Geometry check sheet. Reference: the model listing, model coordinates, mm. Round coordinates to 2 decimals unless told otherwise and drop trailing zeros. Write each loop counter-clockwise with the first axis right and the second up, starting at its lowest first coordinate (ties: lowest second). Pieces come first, ordered by that corner, then holes. Notation, with made-up numbers: (-35, 36.5) -> (-29, 36.5) arc R16 ccw to (-29, 66.5) -> close; hole circle Ø7 at (-27, 69.25). An arc over 180 degrees is marked (long way). One line per question, with ' | ' between items.
```python
from build123d import *

# Parameters (mm, degrees)
EXTRUDE_THIN1_START = 1
EXTRUDE_THIN1_DEPTH = 6.35


with BuildPart() as part:
    # Sketch1 → Extrude-Thin1 (new body)
    with BuildSketch(Plane.XY.offset(EXTRUDE_THIN1_START)):
        with BuildLine():
            Line((388.165618503, 2.23097434), (388.165618503, 5.41097434))
            ThreePointArc((388.165618503, 5.41097434), (388.136623681, 5.481389287), (388.066453208, 5.510970857))
            Line((388.066453208, 5.510970857), (0.059901443, 8.749794959))
            ThreePointArc((0.059901443, 8.749794959), (-8.749999578, 0.002718342), (0.054464874, -8.749830488))
            Line((0.054464874, -8.749830488), (487.776522402, -5.713917899))
            ThreePointArc((487.776522402, -5.713917899), (493.304398035, -0.153253749), (487.779978506, 5.410843992))
            Line((487.779978506, 5.410843992), (428.265786749, 5.510974199))
            ThreePointArc((428.265786749, 5.510974199), (428.194967334, 5.481744477), (428.165618503, 5.41097434))
            Line((428.165618503, 5.41097434), (428.165618503, 2.23097434))
            Line((428.165618503, 2.23097434), (427.665618503, 2.23097434))
            Line((427.665618503, 2.23097434), (427.665618503, 5.41097434))
            ThreePointArc((427.665618503, 5.410974341), (427.841711488, 5.835595162), (428.266627977, 6.010973491))
            Line((428.266627977, 6.010973491), (487.78208283, 5.91084116))
            ThreePointArc((487.78208283, 5.91084116), (493.804398179, -0.15274976), (487.77963468, -6.213908213))
            Line((487.77963468, -6.213908213), (0.057577153, -9.249820802))
            ThreePointArc((0.057577153, -9.249820802), (-9.249999493, 0.003063934), (0.063704889, 9.249780629))
            Line((0.063704889, 9.249780629), (388.070626735, 6.010953438))
            ThreePointArc((388.070626735, 6.010953438), (388.491649569, 5.833464021), (388.665618503, 5.410974341))
            Line((388.665618503, 5.410974341), (388.665618503, 2.23097434))
            Line((388.665618503, 2.23097434), (388.165618503, 2.23097434))
        make_face()
    extrude(amount=EXTRUDE_THIN1_DEPTH)


solid = part.part
```
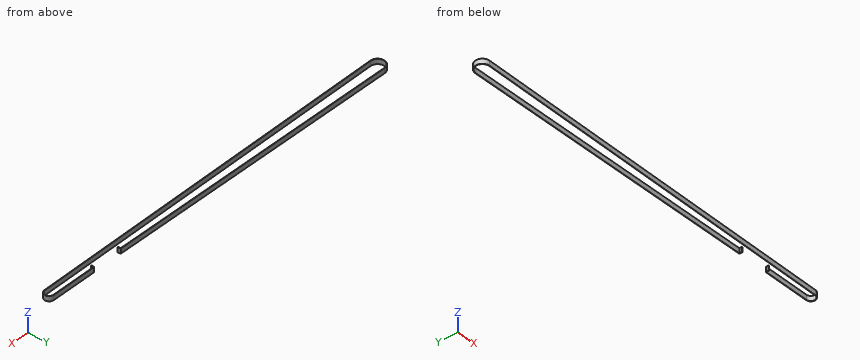
(1) Go/stop test with flat-tipped pins: pin 1 (0.6 mm diameter, centred on x = 428, z = 3.5, fed in from -Y); pin 2 (1 mm diameter, centred on y = -5, z = 4, fed in from -X); pin 3 (1.6 mm diameter, centred on y = 3, z = 5, fed in from +X). Record where each tip stops, or that it passes through.
Resolved:
pin 1: stops at y = -6.59 | pin 2: stops at x = -8.08 | pin 3: stops at x = 493.33
(2) Material ranges on line 1 (X direction, y = -1, z = 4); line 2 (X direction, y = 2.5, z = 5.25); line 3 (X direction, y = -0.75, z = 5.25), recorded low to high.
Resolved:
line 1: x = -9.2 to -8.69, 493.24 to 493.74 | line 2: x = -8.91 to -8.39, 388.17 to 388.67, 427.67 to 428.17, 492.63 to 493.19 | line 3: x = -9.22 to -8.72, 493.27 to 493.77
(3) Sectioned sample at B-B on x = 358.5. Record the cut outline in (y, z).
Resolved:
outline: (-7.02, 1) -> (-6.52, 1) -> (-6.52, 7.35) -> (-7.02, 7.35) -> close; (5.76, 1) -> (6.26, 1) -> (6.26, 7.35) -> (5.76, 7.35) -> close
